Verification items for this drawing (mm, ordinates from the low corner). A direction names the side the tool comes from. Round coordinates to 2 decimals unless told otherwise and drop trailing zeros. Write each loop counter-clockwise with the first axis right and the second up, starting at its lowest first coordinate (ties: lowest second). Pieces come first, ordered by that corner, then holes. Notation, with made-up numbers: (-28, -32) -> (29, -32) arc R24 cw to (29, 7) -> close; hole circle Ø9 at (45.5, -18). An arc over 180 degrees is marked (long way). One line per question, with ' | ' between items.
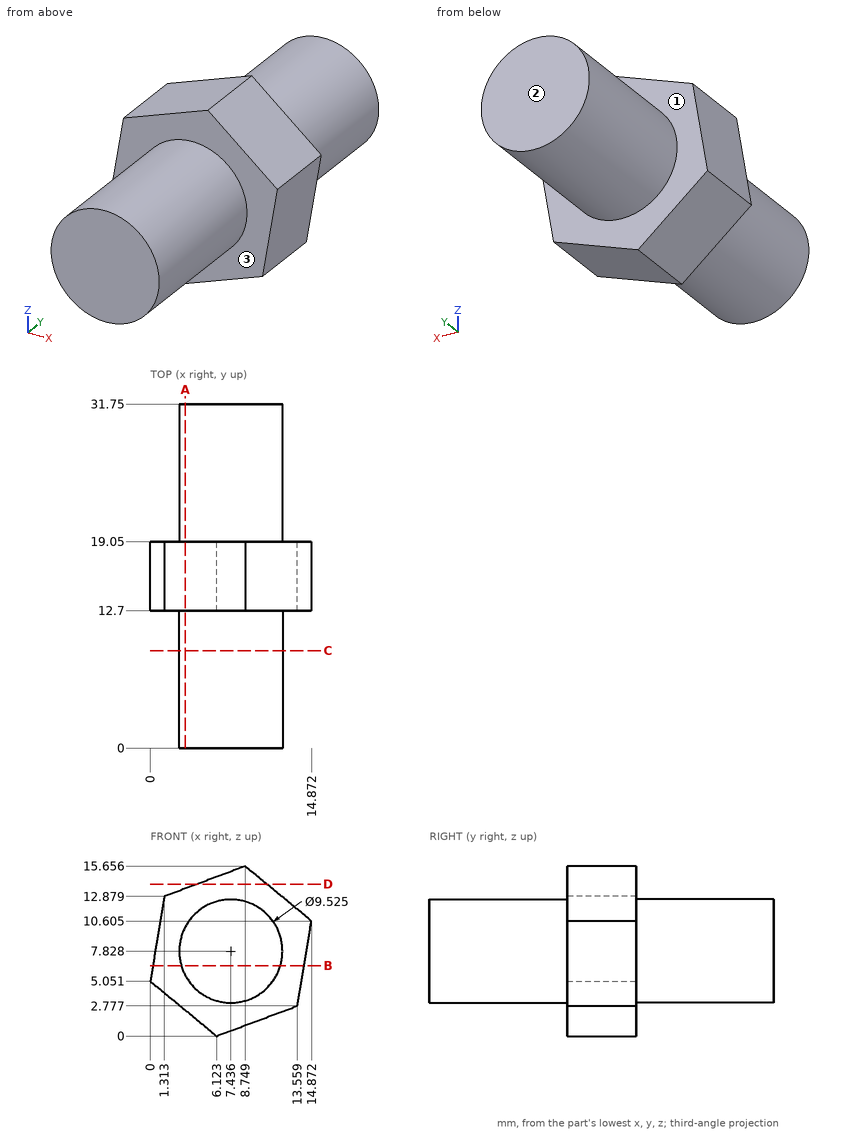
(1) Go/stop test with flat-tipped pins: pin 1 (3 mm diameter, centred on y = 15.5, z = 5.5, fed in from +X); pin 2 (8 mm diameter, centred on y = 19.5, z = 13.5, fed in from -X); pin 3 (6 mm diameter, centred on y = 15, z = 7, fed in from -X). Record where each tip stops, or that it passes through.
Resolved:
pin 1: stops at x = 14.27 | pin 2: stops at x = 0.75 | pin 3: stops at x = 0
(2) Sectioned sample at A-A on x = 3.25. Record the cut outline in (y, z).
Resolved:
outline: (0, 5.56) -> (12.7, 5.56) -> (12.7, 2.37) -> (19.05, 2.37) -> (19.05, 5.56) -> (31.75, 5.56) -> (31.75, 10.1) -> (19.05, 10.1) -> (19.05, 13.6) -> (12.7, 13.6) -> (12.7, 10.1) -> (0, 10.1) -> close
(3) Sectioned sample at C-C on y = 9. Record the cut outline in (x, z) (1 decimal).
Resolved:
outline: circle Ø9.5 at (7.4, 7.8)
(4) Material ranges on line 1 (Z direction, x = 7.5, y = 23); line 2 (Y direction, x = 10.25, z = 14.25); line 3 (X direction, y = 15.5, z = 5.25), recorded low to high.
Resolved:
line 1: z = 3.07 to 12.59 | line 2: y = 12.7 to 19.05 | line 3: x = 0.03 to 13.97
(5) Access from +Z, -Z, +X, -X, +Y, -Y to the whole of each face (thin tool, end or side, straight path). Record for the marked faces 1, 2 and 3.
Resolved:
face 1: +Y | face 2: +Z, -Z, +X, -X, +Y | face 3: -Y
(6) Sectioned sample at D-D on z = 14. Record the cut outline in (x, y).
Resolved:
outline: (4.31, 12.7) -> (10.76, 12.7) -> (10.76, 19.05) -> (4.31, 19.05) -> close
(7) Sectioned sample at B-B on z = 6.5. Record the cut outline in (x, y), then the cut area to 3 significant figures.
Resolved:
outline: (0.24, 12.7) -> (2.86, 12.7) -> (2.86, 0) -> (12.01, 0) -> (12.01, 12.7) -> (14.18, 12.7) -> (14.18, 19.05) -> (12.01, 19.05) -> (12.01, 31.75) -> (2.86, 31.75) -> (2.86, 19.05) -> (0.24, 19.05) -> close | area: 321 mm2
